Study the drawing (mm; zero at the part's minimum x, y, z) and answer. Round coordinates to 2 decimals unless told otherwise and drop trailing zeros. Loops run counter-clockwise (first coordinate to the right, second up) from the corner with the lowest first, then second, coordinate; pieces in that order, holes last. Notation, with made-up numbers: M -25.75,-15.75 L -21.75,-15.75 A36 cw -21.75,19.25 Z; hole C 25.25,49 d5. An arc over 180 degrees is marked long. Put each result on its own line as item: value. Start each with the question number.
(1) Determine the mould class of the marked faces 1, 2, 3 and 4 for opening direction X: released by +X, released by -X, zero draft, split by the parting line, or undercut.
(2) Straight lines are drawn through the part: line 1 (Y direction, x = 5, z = 2.75); line 2 (X direction, y = 6.75, z = 2.1). For each, find the intervals that lie inside material, in ascending order.
(3) Section B-B, the plane y = 5 is taken. Determine the outline of the cut face in (x, z) (3 decimals).
(4) Section D-D, the plane z = 0.4 is taken. Determine the outline of the cut face in (x, y) (3 decimals), then the cut area to 3 significant figures.
(5) Section A-A, the plane z = 4.3 is taken. Determine the outline of the cut face in (x, y), then the cut area to 3 significant figures.
(6) Flat-ended cylindrical pins translate along their axes: P1, Ø1, axis at x = 5, z = 3.5, coming from the -Y side; P2, Ø6, axis at x = 5, y = 5, coming from the +Z side (3 decimals). Find the tip coordinate at first contact, or state that the pin passes through.
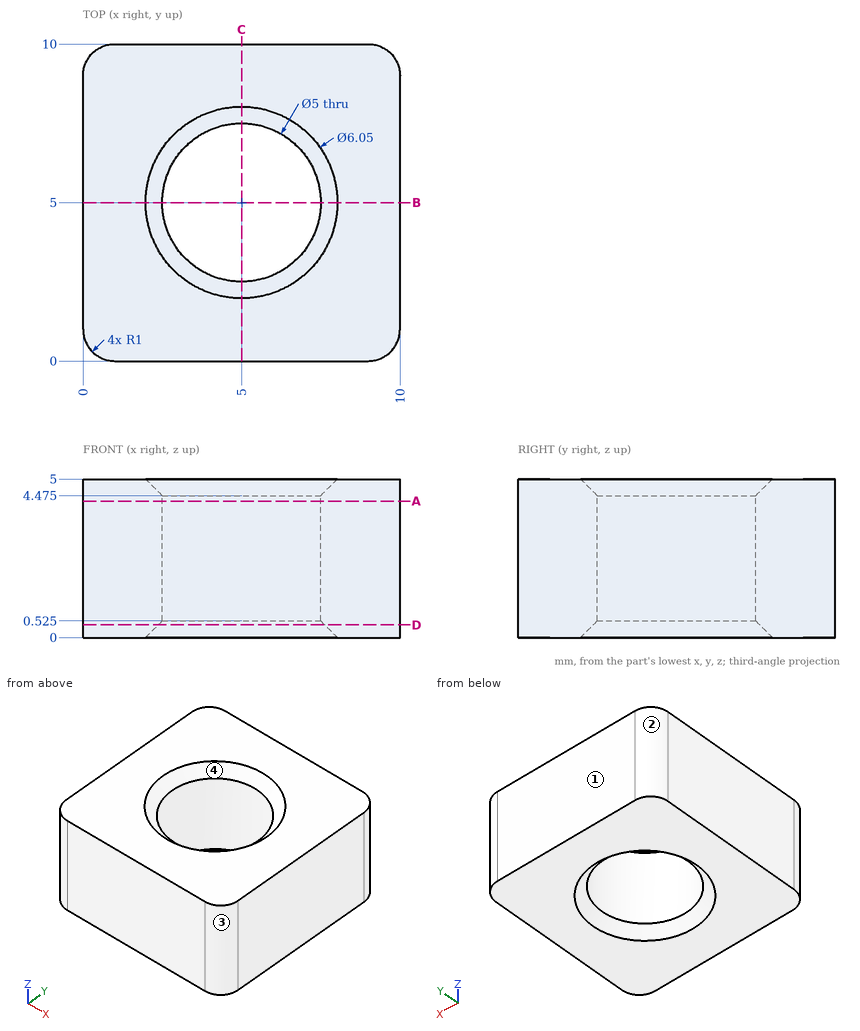
Recorded:
1. face 1: zero draft
1. face 2: released by -X
1. face 3: released by +X
1. face 4: undercut
2. line 1: y = 0 to 2.5, 7.5 to 10
2. line 2: x = 0 to 3.21, 6.79 to 10
3. outline: M 0,0 L 1.975,0 L 2.5,0.525 L 2.5,4.475 L 1.975,5 L 0,5 Z; M 7.5,0.525 L 8.025,0 L 10,0 L 10,5 L 8.025,5 L 7.5,4.475 Z
4. outline: M 0,1 A1 ccw 1,0 L 9,0 A1 ccw 10,1 L 10,9 A1 ccw 9,10 L 1,10 A1 ccw 0,9 Z; hole C 5,5 d5.25
4. area: 77.5 mm²
5. outline: M 0,1 A1 ccw 1,0 L 9,0 A1 ccw 10,1 L 10,9 A1 ccw 9,10 L 1,10 A1 ccw 0,9 Z; hole C 5,5 d5
5. area: 79.5 mm²
6. P1: stops at y = 0
6. P2: stops at z = 4.975
